Build history of the part. All positions in model axes, mm. Face numbers are marked on the shaded views. A direction names the side the tool comes from. Round coordinates to 2 decimals unless told otherwise and drop trailing zeros. Write each loop counter-clockwise with the first axis right and the second up, starting at its lowest first coordinate (ties: lowest second). Pieces come first, ordered by that corner, then holes.
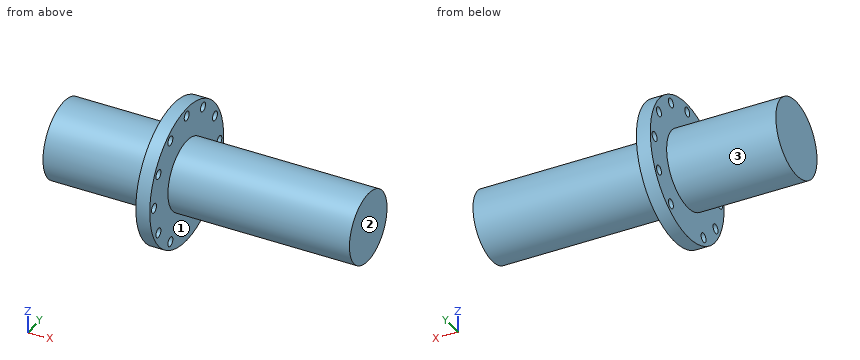
from build123d import *

# Parameters (mm, degrees)
M6_CLEARANCE_HOLE1_D = 6.6


with BuildPart() as part:
    # Sketch1 → Revolve1 (revolve)
    with BuildSketch(Plane(origin=(0, 0, 0), x_dir=(1, 0, 0), z_dir=(0, 1, 0)), mode=Mode.PRIVATE) as revolve1_sk:
        Polygon((0, 0), (215, 0), (215, 25.019), (148.198, 25.019), (86.8925, 25.019), (86.8925, 49.25), (77.05, 49.25), (77.05, 27.432), (0, 27.432), align=None)
    revolve(revolve1_sk.sketch.rotate(Axis((0, 0, 0), (1, 0, 0)), 180), axis=Axis((0, 0, 0), (1, 0, 0)))

    # M6 Clearance Hole1 (through all)
    with Locations(Plane(origin=(77.05, -25.41686526, -173.860891127), x_dir=(0, 0.3426508024612423, 0.9394628399104814), z_dir=(-1, 0, 0))):
        with Locations((129.200757828, -43.220313279), (138.703261819, -63.634261455), (157.139645763, -76.562007172), (179.56989547, -78.539571404), (199.983843646, -69.037067413), (212.911589362, -50.60068347), (214.889153595, -28.170433763), (205.386649604, -7.756485587), (186.95026566, 5.17126013), (164.520015953, 7.148824362), (144.106067777, -2.353679629)):
            Hole(M6_CLEARANCE_HOLE1_D / 2)


solid = part.part
1) Slice it at A-A (z = 0). Write the cut outline in (x, y).
Results:
outline: (0, -27.43) - (77.05, -27.43) - (77.05, -40.2) - (86.89, -40.2) - (86.89, -25.02) - (215, -25.02) - (215, 25.02) - (86.89, 25.02) - (86.89, 40.2) - (77.05, 40.2) - (77.05, 27.43) - (0, 27.43) - close; (77.05, -49.25) - (86.89, -49.25) - (86.89, -46.8) - (77.05, -46.8) - close; (77.05, 46.8) - (86.89, 46.8) - (86.89, 49.25) - (77.05, 49.25) - close
2) Slice it at D-D (x = 119.5). Write the cut outline in (y, z), plus the area to 3 significant figures.
Results:
outline: circle Ø50.04 at (0, 0)
area: 1,970 mm2
3) Which spindle directions (+Z, -Z, +X, -X, +Y, -Y) get a long thin tool onto all of the face, cutting with end or side? Do the marked faces 1, 2 and 3. Say none if no direction does.
Results:
face 1: +X
face 2: +Z, -Z, +X, +Y, -Y
face 3: -X
4) Slice it at B-B (z = 43.5). Write the cut outline in (x, y), plus the area to 3 significant figures.
Results:
outline: (77.05, -23.09) - (86.89, -23.09) - (86.89, -3.3) - (77.05, -3.3) - close; (77.05, 3.3) - (86.89, 3.3) - (86.89, 23.09) - (77.05, 23.09) - close
area: 390 mm2
5) Slice it at C-C (y = 14). Write the cut outline in (x, z), plus the area to 3 significant figures.
Results:
outline: (0, -23.59) - (77.05, -23.59) - (77.05, -47.22) - (86.89, -47.22) - (86.89, -20.74) - (215, -20.74) - (215, 20.74) - (86.89, 20.74) - (86.89, 47.22) - (77.05, 47.22) - (77.05, 23.59) - (0, 23.59) - close
area: 9,880 mm2
6) Pin check, flat tips, straight feed: pin 1 Ø8.5 at (y, z) = (-21.75, -37.67) entering from +X; pin 2 Ø6 at (x, z) = (35, 13) entering from +Y; pin 3 Ø6 at (y, z) = (37.67, 21.75) entering from -X; pin 4 Ø10 at (x, z) = (166, 11) entering from +Y. Stop position of each tip, or through.
Results:
pin 1: stops at x = 86.89
pin 2: stops at y = 25.54
pin 3: passes through
pin 4: stops at y = 24.29
7) Wall check: L1, parallel to Y at x = 84, z = 0; L2, parallel to Y at x = 81, z = -21.75; L3, parallel to X at y = 12, z = -29. Give the ranges that are in metal, low to high.
Results:
L1: y = -49.25 to -46.8, -40.2 to 40.2, 46.8 to 49.25
L2: y = -44.19 to -40.97, -34.37 to 34.37, 40.97 to 44.19
L3: x = 77.05 to 86.89
